Work out the finished part from the listing and answer in its coordinate system (mm). A direction names the side the tool comes from. Coordinates: 2 decimals unless noted, no trailing zeros. Order: outer loops, then holes, each group sorted by start corner. A loop starts at its lowest first (then second) coordinate and runs counter-clockwise, first axis right, second up. Notation, with made-up numbers: (1.25, 44.5) -> (9.25, 44.5) arc R23 cw to (9.25, 68.5) -> close; hole circle Ø5 at (11.5, 3.25). An arc over 180 degrees is marked (long way). Use one line per item in the form item = value.
Autodesk Inventor part; units mm, degrees
ref_plane "YZ Plane" through (0, 0, 0) normal (1, 0, 0) x (0, 1, 0)
ref_plane "XZ Plane" through (0, 0, 0) normal (0, 1, 0) x (-1, 0, 0)
ref_plane "XY Plane" through (0, 0, 0) normal (0, 0, 1) x (1, 0, 0)
sketch "Sketch1" plane through (0, 0, 0) normal (0, 0, 1) x (1, 0, 0)
  circle A0 centre (0, 0) radius 4.5
  circle A1 centre (0, 0) radius 6
  dimension "d0" = 9
  dimension "d1" = 12
extrude "Extrusion1" add sketch "Sketch1" along normal blind 15
chamfer "Chamfer1" distance 0.5 angle 45 2 edges at (-6, 0, 15) (-6, 0, 0)
sketch "Sketch2" plane through (0, 0, 0) normal (1, 0, 0) x (0, 1, 0)
  circle A0 centre (0, 11.4223) radius 1.5
  circle A1 centre (0, 4.4743) radius 1.5
  point P0 (0, 0)
  dimension "d7" = 3
  dimension "d8" = 3
extrude "Extrusion2" cut sketch "Sketch2" against normal blind 10
thread "Thread1"
thread "Thread2"
equation "\"BendRadius\" = Thickness"
equation "\"BendReliefWidth\" = Thickness"
equation "\"BendReliefDepth\" = 0.5 * Thickness"
equation "\"CornerReliefSize\" = 4 * Thickness"
equation "\"MinimumRemnant\" = 2 * Thickness"
equation "\"TransitionRadius\" = BendRadius"
equation "\"JacobiRadiusSize\" = BendRadius"
equation "\"GapSize\" = Thickness"
properties part number "khớp nối"
(1) Straight lines are drawn through the part: line 1 along Y through (x, z) = (0, 12.5); line 2 along Y through (x, z) = (3.25, 1); line 3 along X through (y, z) = (0, 11.75). For each, find the intervals that lie inside material, in ascending order.
Data:
line_1 = -6 to -4.5, 4.5 to 6
line_2 = -5.04 to -3.11, 3.11 to 5.04
line_3 = 4.5 to 6
(2) The mould has two halves that part along Y. Classify faces 1 (the cylindrical face through (-5.109, 0.806, 12.687)), 2 (the flat face through (-5, 0, 0)), 3 (the cylindrical face through (5.723, -1.802, 7.402)): released by +Y, released by -Y, zero draft, split by the parting line, or undercut.
Data:
face_1 = undercut
face_2 = zero draft
face_3 = split by the parting line
(3) Section A-A on y = 0 is taken. Write down the section's boundary in (x, z).
Data:
outline = (-6, 0.5) -> (-5.5, 0) -> (-4.5, 0) -> (-4.5, 2.97) -> (-6, 2.97) -> close; (-6, 5.97) -> (-4.5, 5.97) -> (-4.5, 9.92) -> (-6, 9.92) -> close; (-6, 12.92) -> (-4.5, 12.92) -> (-4.5, 15) -> (-5.5, 15) -> (-6, 14.5) -> close; (4.5, 0) -> (5.5, 0) -> (6, 0.5) -> (6, 14.5) -> (5.5, 15) -> (4.5, 15) -> close
(4) Section C-C on z = 9.25 is taken. Write down the section's boundary in (x, y), plus the area to 3 significant figures.
Data:
outline = circle Ø12 at (0, 0); hole circle Ø9 at (0, 0)
area = 49.5 mm²
(5) Each of these flat-tipped pins is pushed along its axis until it touches: P1, Ø1, axis at y = -2, z = 11.5, coming from the +X side; P2, Ø5, axis at y = 1, z = 6, coming from the +X side. Where does it stop, or does it pass through?
Data:
P1 = 5.81
P2 = 6
(6) Section B-B on x = 0 is taken. Write down the section's boundary in (y, z), plus the area to 3 significant figures.
Data:
outline = (-6, 0.5) -> (-5.5, 0) -> (-4.5, 0) -> (-4.5, 15) -> (-5.5, 15) -> (-6, 14.5) -> close; (4.5, 0) -> (5.5, 0) -> (6, 0.5) -> (6, 14.5) -> (5.5, 15) -> (4.5, 15) -> close
area = 44.5 mm²
(7) Which of the six approach directions +Z, -Z, +X, -X, +Y, -Y give full straight-line access (tool end or side, diameter ignored) to faces 4 (the cylindrical face through (-5.109, 1.431, 4.925)), 5 (the flat face through (-5, 0, 15))?
Data:
face_4 = -X
face_5 = +Z, +X, -X, +Y, -Y
(8) Section D-D on z = 5.75 is taken. Write down the section's boundary in (x, y).
Data:
outline = (-5.95, -0.79) arc R6 ccw (long way) to (-5.95, 0.79) -> (-4.43, 0.79) arc R4.5 cw (long way) to (-4.43, -0.79) -> close
